The listing builds one solid part. Answer for the finished solid, in the listing's coordinates (mm). A direction names the side the tool comes from. Coordinates: 2 decimals unless noted, no trailing zeros. Loops run counter-clockwise (first coordinate to the right, second up) from the corner with the lowest first, then second, coordinate; pieces in that order, holes last. Notation, with made-up numbers: (-23.5, 82.5) - (1.5, 82.5) arc R20 ccw to (1.5, 86.5) - close; hole circle Ø3 at (30.25, 76.25). An arc over 180 degrees is marked (long way). Use one line per item in the form item = value. Start each with the question number.
```python
from build123d import *

# Parameters (mm, degrees)
SKETCH1_R           = 9.6
BOSS_EXTRUDE1_DEPTH = 72
SKETCH2_R           = 2.6
CUT_EXTRUDE1_DEPTH  = 6
CHAMFER1_SIZE       = 0.5
CHAMFER2_SIZE       = 1


with BuildPart() as part:
    # Sketch1 → Boss-Extrude1 (new body)
    with BuildSketch(Plane(origin=(0, 0, 0), x_dir=(1, 0, 0), z_dir=(0, 1, 0))):
        with BuildLine():
            Line((14.966629547, 3), (16, 3))
            Line((16, 3), (16, 11))
            Line((16, 11), (-16, 11))
            Line((-16, 11), (-16, 3))
            Line((-16, 3), (-14.966629547, 3))
            ThreePointArc((-14.966629547, 3), (-13.50603606, 2.366260102), (-12.971078941, 0.866666667))
            ThreePointArc((-12.971078941, 0.866666667), (0, -13), (12.971078941, 0.866666667))
            ThreePointArc((12.971078941, 0.866666667), (13.50603606, 2.366260102), (14.966629547, 3))
        make_face()
        with Locations(Location((0, 0, 0), (0, 0, 270))):  # turned: the seam where the file's is
            Circle(SKETCH1_R, mode=Mode.SUBTRACT)
    extrude(amount=BOSS_EXTRUDE1_DEPTH)

    # Sketch2 → Cut-Extrude1 (cut)
    with BuildSketch(Plane.XY.offset(-11)):
        with Locations((-11, 67)):
            Circle(SKETCH2_R)
        with Locations((-11, 5)):
            Circle(SKETCH2_R)
        with Locations((11, 67)):
            Circle(SKETCH2_R)
        with Locations((11, 5)):
            Circle(SKETCH2_R)
    extrude(amount=CUT_EXTRUDE1_DEPTH, mode=Mode.SUBTRACT)

    # Chamfer1
    chamfer1_edges = [part.edges().sort_by_distance(p)[0] for p in [
        (-13.6, 67, -11),
        (-13.6, 5, -11),
        (8.4, 67, -11),
        (8.4, 5, -11),
    ]]
    chamfer(chamfer1_edges, length=CHAMFER1_SIZE)

    # Chamfer2
    chamfer2_edges = [part.edges().sort_by_distance(p)[0] for p in [
        (0, 0, -9.6),
        (0, 72, -9.6),
    ]]
    chamfer(chamfer2_edges, length=CHAMFER2_SIZE)


solid = part.part
```
(1) A cutting plane is placed at B-B (y = 30). Determine the outline of the cut face in (x, z), then the cut area to 3 significant figures.
(2) A cutting plane is placed at D-D (y = 5). Determine the outline of the cut face in (x, z).
(3) A cutting plane is placed at C-C (z = -7.5). State how many separate pieces and enclosed holes the cut face has, then the cut area to 3 significant figures.
(4) Each of these flat-tipped pins is pushed along its axis until it touches: pin 1 Ø2.5 at (x, y) = (12, 4) entering from -Z; pin 2 Ø0.5 at (x, y) = (15.5, 45) entering from +Z; pin 3 Ø3 at (x, y) = (-10.5, 26.5) entering from +Z; pin 4 Ø5.5 at (x, y) = (12, 67.5) entering from -Z. Where does it stop, or does it pass through?
(5) For faces 1 (the face through (11, 5, -5)), 2 (the face through (0, 35, -11)), determine the directions among +Z, -Z, +X, -X, +Y, -Y from which every point of the face is accessible in a straight line to the end or side of a thin tool.
(6) Determine the mould class of faces 3 (the face through (9.4, 72, -5.3)), 4 (the face through (0, 35, 13)), 5 (the face through (11, 67, -5)) for opening direction Y: +Y half, -Y half, draft (parallel to the pull), parting line (faces both ways), or undercut.
(7) Find the intervals of material crossed by probe 1 along Y at (x, z) = (-11, -7.7); probe 2 along X at (y, z) = (55, 0); probe 3 along X at (y, z) = (33, 6), in increasing order. Write a range as from..to.
(8) A cutting plane is placed at A-A (z = 0). Determine the outline of the cut face in (x, y).
Evaluation:
q1.outline = (-16, -11) - (16, -11) - (16, -3) - (14.97, -3) arc R2 cw to (12.97, -0.87) arc R13 ccw (long way) to (-12.97, -0.87) arc R2 cw to (-14.97, -3) - (-16, -3) - close; hole circle Ø19.2 at (0, 0)
q1.area = 311 mm^2
q2.outline = (-16, -11) - (-14.1, -11) - (-13.6, -10.5) - (-13.6, -5) - (-8.4, -5) - (-8.4, -10.5) - (-7.9, -11) - (7.9, -11) - (8.4, -10.5) - (8.4, -5) - (13.6, -5) - (13.6, -10.5) - (14.1, -11) - (16, -11) - (16, -3) - (14.97, -3) arc R2 cw to (12.97, -0.87) arc R13 ccw (long way) to (-12.97, -0.87) arc R2 cw to (-14.97, -3) - (-16, -3) - close; hole circle Ø19.2 at (0, 0)
q3.separate_pieces = 2
q3.enclosed_holes = 4
q3.area = 1,350 mm^2
q4.pin_1 = -10.56
q4.pin_2 = -3
q4.pin_3 = 9.38
q4.pin_4 = -11
q5.face_1 = -Z
q5.face_2 = -Z, +X, -X, +Y, -Y
q6.face_3 = +Y half
q6.face_4 = draft
q6.face_5 = undercut
q7.probe_1 = 0..2.4, 7.6..64.4, 69.6..72
q7.probe_2 = -13..-9.6, 9.6..13
q7.probe_3 = -11.53..-7.49, 7.49..11.53
q8.outline = (-13, 0) - (-10.6, 0) - (-9.6, 1) - (-9.6, 71) - (-10.6, 72) - (-13, 72) - close; (9.6, 1) - (10.6, 0) - (13, 0) - (13, 72) - (10.6, 72) - (9.6, 71) - close
